from build123d import *

# Parameters (mm, degrees)
EXTRUDE_1_DEPTH     = 59
SKETCH_2_R          = 4.25
CUT_EXTRUDE_1_DEPTH = 9
SKETCH_3_R          = 4.25
CUT_EXTRUDE_2_DEPTH = 9


with BuildPart() as part:
    # Эскиз1 → Бобышка-Вытянуть1 (new body, symmetric)
    with BuildSketch(Plane.XY):
        Polygon((-78, 0), (0, 0), (0, 78), (-8, 78), (-8, 68.5), (-7.5, 68), (-8, 67.5), (-8, 54.5), (-7.5, 54), (-8, 53.5), (-8, 40.5), (-7.5, 40), (-8, 39.5), (-8, 30), (-30, 8), (-39.5, 8), (-40, 7.5), (-40.5, 8), (-53.5, 8), (-54, 7.5), (-54.5, 8), (-67.5, 8), (-68, 7.5), (-68.5, 8), (-78, 8), align=None)
        with BuildLine():
            Line((-4.5, 12), (-4.5, 26.136038969))
            ThreePointArc((-4.5, 26.136038969), (-5.117316568, 27.059918502), (-6.207106781, 26.843145751))
            Line((-6.207106781, 26.843145751), (-26.843145751, 6.207106781))
            ThreePointArc((-26.843145751, 6.207106781), (-27.059918502, 5.117316568), (-26.136038969, 4.5))
            Line((-26.136038969, 4.5), (-12, 4.5))
            Line((-12, 4.5), (-12, 7.9))
            ThreePointArc((-12, 7.9), (-14.899137803, 9.100862197), (-16.1, 12))
            ThreePointArc((-16.1, 12), (-15.1, 13), (-14.1, 12))
            ThreePointArc((-14.1, 12), (-10.51507576, 10.51507576), (-12, 14.1))
            ThreePointArc((-12, 14.1), (-13, 15.1), (-12, 16.1))
            ThreePointArc((-12, 16.1), (-9.100862197, 14.899137803), (-7.9, 12))
            Line((-7.9, 12), (-4.5, 12))
        make_face(mode=Mode.SUBTRACT)
    extrude(amount=EXTRUDE_1_DEPTH, both=True)

    # Эскиз2 → Вырез-Вытянуть1 (cut, through all)
    with BuildSketch(Plane.ZY.offset(8)):
        with Locations(Location((-40, 54, 0), (0, 0, 270))):  # turned: the seam where the file's is
            Circle(SKETCH_2_R)
        with Locations(Location((40, 54, 0), (0, 0, 270))):  # turned: the seam where the file's is
            Circle(SKETCH_2_R)
    extrude(amount=-CUT_EXTRUDE_1_DEPTH, mode=Mode.SUBTRACT)

    # Эскиз3 → Вырез-Вытянуть2 (cut, through all)
    with BuildSketch(Plane(origin=(0, 8, 0), x_dir=(1, 0, 0), z_dir=(0, 1, 0))):
        with Locations(Location((-54, -40, 0), (0, 0, 180))):  # turned: the seam where the file's is
            Circle(SKETCH_3_R)
        with Locations(Location((-54, 40, 0), (0, 0, 180))):  # turned: the seam where the file's is
            Circle(SKETCH_3_R)
    extrude(amount=-CUT_EXTRUDE_2_DEPTH, mode=Mode.SUBTRACT)


solid = part.part
Design review of the part built by this model. Coordinates are the model's own, in mm. A direction names the side the tool comes from. Coordinates: 2 decimals unless noted, no trailing zeros. Loops run counter-clockwise (first coordinate to the right, second up) from the corner with the lowest first, then second, coordinate; pieces in that order, holes last. Notation, with made-up numbers: (39.25, -9) - (72.25, -9) arc R23 cw to (72.25, 11) - close; hole circle Ø6 at (55, -29.5). An arc over 180 degrees is marked (long way). Use CSV: the item, a comma, the result in double quotes. Start each with the question number.
1. Add section B-B on z = 40. Count the separate pieces of the cut face and the enclosed holes in it, plus the area to 3 significant figures.
2. Add section A-A on x = -20.5. Give the boundary of the cut face in (y, z), plus the area to 3 significant figures.
3. Clearance check with flat-ended pins moving along their axes: pin 1 (14.5 mm diameter, centred on x = -63, z = 20.5, fed in from +Y); pin 2 (11 mm diameter, centred on y = 54, z = 40, fed in from -X); pin 3 (10 mm diameter, centred on x = -15, y = 69, fed in from +Z); pin 4 (3 mm diameter, centred on x = -11, z = 2, fed in from +Y). State where each tip first meets the part, or that it passes through.
4. To check wall thickness, follow probe 1 along Z at (x, y) = (-5, 54); probe 2 along Y at (x, z) = (-3, 40); probe 3 along X at (y, z) = (15, -41.5). State the ranges of each line that lie inside material, in increasing order.
5. Mouldability with a two-part tool opening along Z and no side actions: class faces 1 (the cylindrical face through (-4.06, 52.04, 36.23)), 2 (the flat face through (-47, 8, 1)), 3 (the flat face through (-19, 16, -59)) as released by +Z, released by -Z, zero draft, split by the parting line, or undercut.
6. Add section D-D on x = -44.5. Give the boundary of the cut face in (y, z).
7. Add section C-C on y = 46.5. Give the boundary of the cut face in (x, z), plus the area to 3 significant figures.
8. For faces 4 (the flat face through (-4.5, 19, 1)), 5 (the flat face through (-4, 78, 1)), 6 (the flat face through (-73, 8, 1)), list the 3-axis set-ups (+Z, -Z, +X, -X, +Y, -Y) from which the entire face can be reached by the end or side of a thin tool; tool diameter is ignored.
Resolved:
1,separate pieces,"3"
1,enclosed holes,"1"
1,area,"1,080 mm2"
2,outline,"(0, -59) - (4.5, -59) - (4.5, 59) - (0, 59) - close; (12.55, -59) - (17.5, -59) - (17.5, 59) - (12.55, 59) - close"
2,area,"1,120 mm2"
3,pin 1,"y = 8"
3,pin 2,"x = -8"
3,pin 3,"through"
3,pin 4,"y = 28.5"
4,probe 1,"-59 to -44.25, -35.75 to 35.75, 44.25 to 59"
4,probe 2,"0 to 49.75, 58.25 to 78"
4,probe 3,"-23 to -18.05, -12.99 to -9.21, -4.5 to 0"
5,face 1,"undercut"
5,face 2,"zero draft"
5,face 3,"released by -Z"
6,outline,"(0, -59) - (8, -59) - (8, 59) - (0, 59) - close"
7,outline,"(-8, -59) - (0, -59) - (0, 59) - (-8, 59) - close"
7,area,"944 mm2"
8,face 4,"+Z, -Z"
8,face 5,"+Z, -Z, +X, -X, +Y"
8,face 6,"+Z, -Z, -X, +Y"
